Could you check a few things on this model? Use its own coordinates, in mm. A direction names the side the tool comes from. Coordinates: 2 decimals unless noted, no trailing zeros. Loops run counter-clockwise (first coordinate to the right, second up) from the corner with the lowest first, then second, coordinate; pieces in that order, holes last. Notation, with made-up numbers: (-20.5, -2.75) - (34.5, -2.75) arc R26 cw to (34.5, 36.25) - close; hole circle Ø3 at (87.25, -13). An arc over 180 degrees is marked (long way). One line per question, with ' | ' between items. Start each with the question number.
1. I'm going to push flat-ended pins straight in: P1, Ø0.8, axis at y = -7, z = 2.5, coming from the +X side; P2, Ø0.8, axis at x = -1, z = 2.5, coming from the -Y side; P3, Ø6, axis at x = -4, y = -7.5, coming from the +Z side. Where does each tip first touch, or does it pass through?
2. Which directions (+Z, -Z, +X, -X, +Y, -Y) give clear straight access to the entire face, cutting with the end or side of a thin tool? Please do faces 1 (the flat face through (0, 2.6, 2)), 2 (the flat face through (0, -2.6, 2)), 3 (the flat face through (0, -8.3, 2)).
3. Please list where these lines run through material, in increasing order: L1, parallel to Y at x = 8.5, z = 1.15; L2, parallel to Z at x = 4, y = -5; L3, parallel to X at y = -7.75, z = 2.55. Write a range as [from, to].
4. I want a section at B-B, the plane x = -8.5. Write out the boundary of the cut face in (y, z), then the cut area to 3 significant figures.
5. We'd pull the mould along X, two halves only. Please class faces 4 (the flat face through (0, 3, 1.6)), 5 (the flat face through (-11.5, 0, 1)), 6 (the cylindrical face through (-8.63, 7.51, 0.79)): pulls with the +X half, pulls with the -X half, needs draft (parallel to the pull), parting line crosses it, or undercut.
6. I want a section at A-A, the plane z = 2.35. Write out the boundary of the cut face in (x, y), then the cut area to 3 significant figures.
7. I want a section at D-D, the plane y = 0.5. Write out the boundary of the cut face in (x, z).
Autodesk Fusion 360 part; units mm, degrees
sketch "Sketch1" plane through (0, 0, 0) normal (0, 0, 1) x (1, 0, 0)
  circle A0 centre (-8.5, 8.5) radius 1
  line L0 (-10.5, 11.5) -> (10.5, 11.5)
  line L1 (11.5, 10.5) -> (11.5, -10.5)
  line L2 (10.5, -11.5) -> (-10.5, -11.5)
  line L3 (-11.5, -10.5) -> (-11.5, 10.5)
  line L4 (-9.5, 11.5) -> (-9.5, 8.5) construction
  line L5 (-7.5, 11.5) -> (-7.5, 8.5) construction
  line L6 (-8.5, 9.5) -> (-11.5, 9.5) construction
  line L7 (0, 11.5) -> (0, -11.5) construction
  line L8 (-11.5, 0) -> (11.5, 0) construction
  circle A1 centre (8.5, 8.5) radius 1
  circle A2 centre (8.5, -8.5) radius 1
  circle A3 centre (-8.5, -8.5) radius 1
  line L9 (-10.5, 11.5) -> (-11.5, 10.5)
  line L10 (10.5, 11.5) -> (11.5, 10.5)
  line L11 (11.5, -10.5) -> (10.5, -11.5)
  line L12 (-10.5, -11.5) -> (-11.5, -10.5)
  point P0 (-11.5, 11.5)
  point P1 (11.5, 11.5)
  point P2 (11.5, -11.5)
  point P3 (-11.5, -11.5)
  dimension "d2" = 23
  dimension "d3" = 23
  dimension "d5" = 2
  dimension "d6" = 19
  dimension "d7" = 2
  dimension "d8" = 1
  dimension "d9" = 1
  dimension "d10" = 1
  dimension "d11" = 1
  dimension "d12" = 1
  dimension "d13" = 1
  dimension "d14" = 1
  dimension "d15" = 1
extrude "Extrude1" add sketch "Sketch1" along normal blind 1.6
sketch "Sketch2" plane through (0, 0, 1.6) normal (0, 0, 1) x (-1, 0, 0)
  circle A0 centre (8.5, 8.5) radius 1
  circle A1 centre (-8.5, -8.5) radius 1
  circle A2 centre (-8.5, 8.5) radius 1
  circle A3 centre (8.5, -8.5) radius 1
  line L0 (10.5, -11.5) -> (11.5, -10.5)
  line L1 (11.5, -10.5) -> (11.5, 10.5)
  line L2 (11.5, 10.5) -> (10.5, 11.5)
  line L3 (10.5, 11.5) -> (-10.5, 11.5)
  line L4 (-10.5, 11.5) -> (-11.5, 10.5)
  line L5 (-11.5, 10.5) -> (-11.5, -10.5)
  line L6 (-11.5, -10.5) -> (-10.5, -11.5)
  line L7 (-10.5, -11.5) -> (10.5, -11.5)
  line L8 (1.9, -2.6) -> (-1.9, -2.6)
  line L9 (-1.9, -2.6) -> (-1.9, 2.6)
  line L10 (-1.9, 2.6) -> (1.9, 2.6)
  line L11 (1.9, 2.6) -> (1.9, -2.6)
  line L12 (11, -11) -> (-11, 11) construction
  line L13 (-11, -11) -> (11, 11) construction
  line L14 (1.9, -2.6) -> (-1.9, 2.6) construction
  line L15 (1.9, 2.6) -> (-1.9, -2.6) construction
  line L16 (6.75, 6.8) -> (-6.75, 6.8)
  line L17 (6.75, 5.3) -> (-6.75, 5.3)
  line L18 (-6.75, 5.3) -> (-6.75, 8.3)
  line L19 (-6.75, 8.3) -> (6.75, 8.3)
  line L20 (6.75, 8.3) -> (6.75, 5.3)
  line L21 (0, 6.8) -> (0, 11.5) construction
  dimension "d18" = 5.2
  dimension "d19" = 3.8
  dimension "d23" = 4.7
  dimension "d24" = 3
  dimension "d25" = 13.5
extrude "Extrude2" add sketch "Sketch2" along normal blind 1.8 contours L8 L9 L10 L11
chamfer "Chamfer1" distance 0.4 angle 45 1 faces at (-0.6333, 0.8667, 3.4)
extrude "Extrude3" add sketch "Sketch2" along normal blind 1.5 contours L16 L17 L18 L20 | L16 L18 L19 L20
sketch "Sketch3" plane through (0, 0, 3.4) normal (0, 0, 1) x (-1, 0, 0)
  line L0 (-1.5, -2.2) -> (1.5, -2.2)
  line L1 (1.5, -2.2) -> (1.5, 2.2)
  line L2 (1.5, 2.2) -> (-1.5, 2.2)
  line L3 (-1.5, 2.2) -> (-1.5, -2.2)
equation "d7 = d5"
equation "d9 = d8"
equation "d11 = d10"
equation "d13 = d12"
equation "d15 = d14"
Results are:
1) P1: stops at x = 6.75 | P2: stops at y = -8.3 | P3: stops at z = 3.1
2) face 1: +Z, +X, -X, +Y | face 2: +Z, +X, -X | face 3: +Z, +X, -X, -Y
3) L1: y = [-11.5, -9.5], [-7.5, 7.5], [9.5, 11.5] | L2: z = [0, 1.6] | L3: x = [-6.75, 6.75]
4) outline: (-11.5, 0) - (-9.5, 0) - (-9.5, 1.6) - (-11.5, 1.6) - close; (-7.5, 0) - (7.5, 0) - (7.5, 1.6) - (-7.5, 1.6) - close; (9.5, 0) - (11.5, 0) - (11.5, 1.6) - (9.5, 1.6) - close | area: 30.4 mm2
5) face 4: needs draft | face 5: pulls with the -X half | face 6: undercut
6) outline: (-6.75, -8.3) - (6.75, -8.3) - (6.75, -5.3) - (-6.75, -5.3) - close; (-1.9, -2.6) - (1.9, -2.6) - (1.9, 2.6) - (-1.9, 2.6) - close | area: 60.3 mm2
7) outline: (-11.5, 0) - (11.5, 0) - (11.5, 1.6) - (1.9, 1.6) - (1.9, 3) - (1.5, 3.4) - (-1.5, 3.4) - (-1.9, 3) - (-1.9, 1.6) - (-11.5, 1.6) - close
